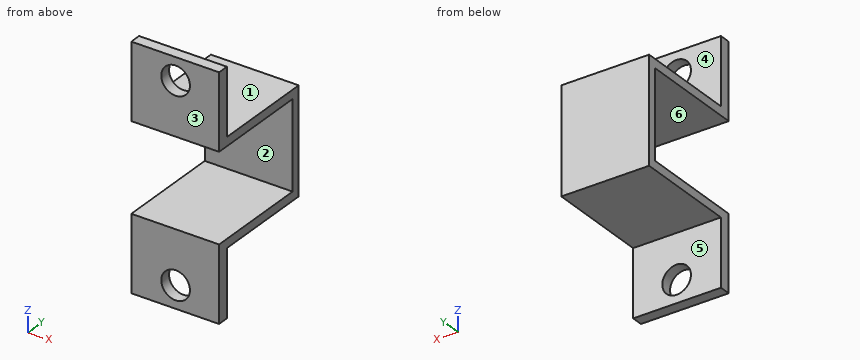
```python
from build123d import *

# Parameters (mm, degrees)
BOSS_EXTRUDE1_DEPTH          = 10
F_30_0_1285_DIAMETER_HOLE1_D = 3.2639


with BuildPart() as part:
    # Sketch1 → Boss-Extrude1 (new body)
    with BuildSketch(Plane(origin=(0, 0, 0), x_dir=(0, 0, -1), z_dir=(1, 0, 0))):
        Polygon((10.828, 0.032), (2.239, 0.032), (2.239, 1.302), (9.828, 1.302), (9.828, 13.032), (14.543, 13.032), (21.828, 13.032), (21.828, 1.302), (29.417, 1.302), (29.417, 0.032), (20.828, 0.032), (20.828, 12.032), (10.828, 12.032), align=None)
    extrude(amount=BOSS_EXTRUDE1_DEPTH)

    # #30 (0.1285) Diameter Hole1 (through all)
    with Locations(Plane(origin=(5.047, 1.302, -26.877), x_dir=(0, 0, 1), z_dir=(0, 1, 0))):
        with Locations((0, 0), (22.098, 0)):
            Hole(F_30_0_1285_DIAMETER_HOLE1_D / 2)


solid = part.part
```
Source: CAD feature listing. Evaluate the final solid. Frame: model axes, mm. Face numbers are marked on the shaded views. A direction names the side the tool comes from. Give positions to 0.01 mm unless a question says otherwise; leave off trailing zeros. Loops run counter-clockwise (first coordinate to the right, second up) from the corner with the lowest first, then second, coordinate; pieces in that order, holes last. Notation, with made-up numbers: (-34.5, 6.25) -> (15.5, 6.25) arc R26 cw to (15.5, 41.25) -> close; hole circle Ø7 at (7, 28.25). An arc over 180 degrees is marked (long way). Use a Markdown table: item, result. Add a question column.
(1) Pull-direction query (Z, two-part tool) for the marked faces 1, 2 and 3; classes: +Z half, -Z half, draft (parallel to the pull), parting line (faces both ways), or undercut.
(2) Section query B-B (z = -25.5). Output: boundary loops of the cut face in (x, y).
(3) Ray query, line 1 (Z direction, x = 7, y = 4); line 2 (Y direction, x = 2, z = -24); line 3 (Y direction, x = 2.5, z = -18.75). Return the intervals inside material, ascending.
(4) Section query C-C (x = 9). Output: boundary loops of the cut face in (y, z), then the cut area to 3 significant figures.
(5) Section query A-A (y = 3.25). Output: boundary loops of the cut face in (x, z).
(6) Access query for the marked faces 4, 5 and 6. Directions: +Z, -Z, +X, -X, +Y, -Y. A direction counts if a zero-diameter tool reaches every point of the face in a straight line with its end or side. Return the directions, or none.
(7) Section query D-D (z = -12.5). Output: boundary loops of the cut face in (x, y).
(8) First-contact query: pin 1 Ø4 at (x, z) = (7, -13.5) entering from -Y; pin 2 Ø2 at (x, y) = (5.5, 10.5) entering from -Z; pin 3 Ø6 at (x, z) = (7, -26) entering from +Y. Flat tips, straight axial feed; report the tip coordinate or a pass-through.
Checked values:
| question | item | result |
|---|---|---|
| 1 | face 1 | +Z half |
| 1 | face 2 | undercut |
| 1 | face 3 | draft |
| 2 | outline | (0, 0.03) -> (4.17, 0.03) -> (4.17, 1.3) -> (0, 1.3) -> close; (5.92, 0.03) -> (10, 0.03) -> (10, 1.3) -> (5.92, 1.3) -> close |
| 3 | line 1 | -21.83 to -20.83, -10.83 to -9.83 |
| 3 | line 2 | 0.03 to 1.3 |
| 3 | line 3 | 12.03 to 13.03 |
| 4 | outline | (0.03, -29.42) -> (1.3, -29.42) -> (1.3, -21.83) -> (13.03, -21.83) -> (13.03, -9.83) -> (1.3, -9.83) -> (1.3, -2.24) -> (0.03, -2.24) -> (0.03, -10.83) -> (12.03, -10.83) -> (12.03, -20.83) -> (0.03, -20.83) -> close |
| 4 | area | 55.3 mm^2 |
| 5 | outline | (0, -21.83) -> (10, -21.83) -> (10, -20.83) -> (0, -20.83) -> close; (0, -10.83) -> (10, -10.83) -> (10, -9.83) -> (0, -9.83) -> close |
| 6 | face 4 | +Z, +X, -X, +Y |
| 6 | face 5 | -Z, +X, -X, +Y |
| 6 | face 6 | +X, -X, -Y |
| 7 | outline | (0, 12.03) -> (10, 12.03) -> (10, 13.03) -> (0, 13.03) -> close |
| 8 | pin 1 | y = 12.03 |
| 8 | pin 2 | z = -21.83 |
| 8 | pin 3 | y = 1.3 |
